from build123d import *

# Parameters (mm, degrees)
SKETCH2_W           = 25
SKETCH2_H           = 10
BOSS_EXTRUDE1_DEPTH = 170
CUT_EXTRUDE1_DEPTH  = 170


with BuildPart() as part:
    # Sketch2 → Boss-Extrude1 (new body)
    with BuildSketch(Plane.XY):
        Rectangle(SKETCH2_W, SKETCH2_H)
    extrude(amount=BOSS_EXTRUDE1_DEPTH)

    # Sketch3 → Cut-Extrude1 (cut)
    with BuildSketch(Plane(origin=(0, 0, 0), x_dir=(-1, 0, 0), z_dir=(0, 0, -1))):
        with BuildLine():
            Line((-8, 5), (8, 5))
            ThreePointArc((8, 5), (0, -3), (-8, 5))
        make_face()
    extrude(amount=-CUT_EXTRUDE1_DEPTH, mode=Mode.SUBTRACT)


solid = part.part
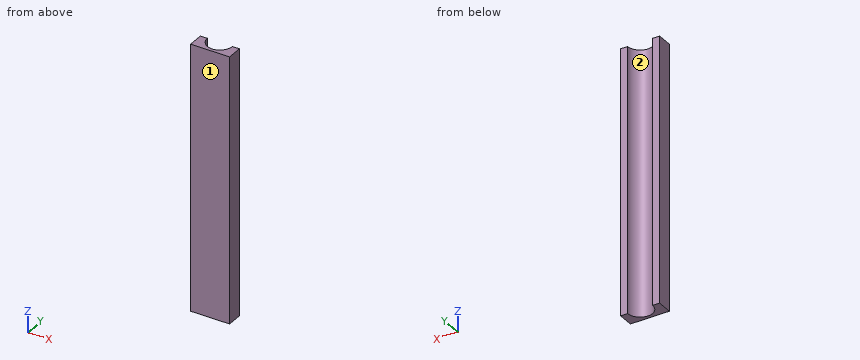
Geometry check sheet. Reference: the model listing, model coordinates, mm. Face numbers are marked on the shaded views. Round coordinates to 2 decimals unless told otherwise and drop trailing zeros. Order: outer loops, then holes, each group sorted by start corner. A loop starts at its lowest first (then second) coordinate and runs counter-clockwise, first axis right, second up. Notation, with made-up numbers: M 14.5,55.25 L 52.5,55.25 A11 cw 52.5,62.25 Z; hole C 45.25,16 d6. An arc over 180 degrees is marked long. Write each question's results on one line, items separated by ' | '. Start each with the question number.
1. Material ranges on L1, parallel to X at y = 4.5, z = 36; L2, parallel to Y at x = -0.5, z = 156; L3, parallel to X at y = 2.5, z = 53, recorded low to high. Write a range as from..to.
2. Draft check along X on the marked faces 1 and 2. Enter one of: pulls with the +X half, pulls with the -X half, needs draft (parallel to the pull), parting line crosses it, or undercut.
3. Cross-section at C-C on x = 0. Record the boundary of the cut face in (y, z), plus the area to 3 significant figures.
4. Cross-section at A-A on y = 0.25. Record the boundary of the cut face in (x, z).
5. Go/stop test with flat-tipped pins: P1, Ø6, axis at x = -3, y = 1.5, coming from the +Z side; P2, Ø12, axis at x = 4.5, z = 131, coming from the +Y side. Record where each tip stops, or that it passes through.
6. Cross-section at B-B on z = 125. Record the boundary of the cut face in (x, y), plus the area to 3 significant figures.
Resolved:
1) L1: -12.5..-7.98, 7.98..12.5 | L2: -5..-2.98 | L3: -12.5..-7.6, 7.6..12.5
2) face 1: needs draft | face 2: undercut
3) outline: M -5,0 L -3,0 L -3,170 L -5,170 Z | area: 340 mm2
4) outline: M -12.5,0 L -6.44,0 L -6.44,170 L -12.5,170 Z; M 6.44,0 L 12.5,0 L 12.5,170 L 6.44,170 Z
5) P1: through | P2: y = 5
6) outline: M -12.5,-5 L 12.5,-5 L 12.5,5 L 8,5 A8 cw -8,5 L -12.5,5 Z | area: 149 mm2
